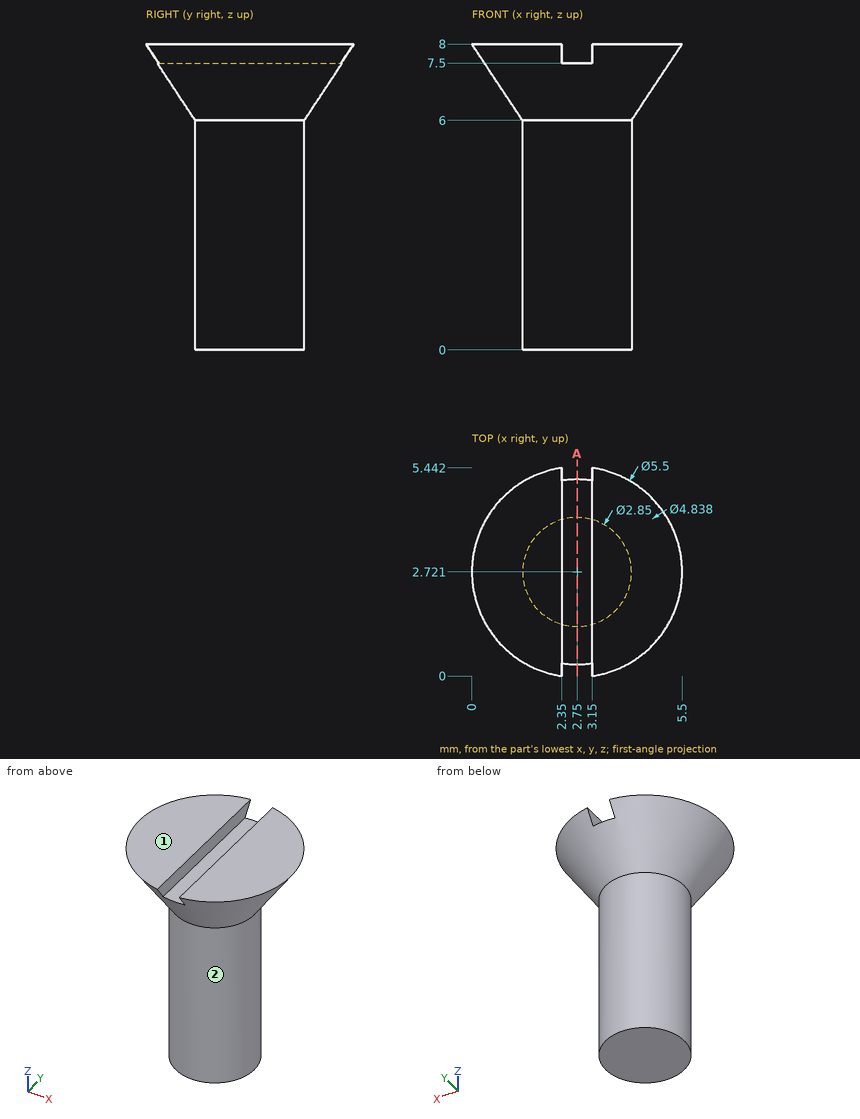
Geometry: see drawing. Coordinates: mm, zero at the bounding-box minimum. A direction names the side the tool comes from. Round coordinates to 2 decimals unless told otherwise and drop trailing zeros. Order: outer loops, then holes, each group sorted by start corner. A loop starts at its lowest first (then second) coordinate and runs counter-clockwise, first axis right, second up. Notation, with made-up numbers: (-34, 86) - (0, 86) arc R26 ccw to (0, 113) - close; hole circle Ø2 at (-32, -12). An arc over 180 degrees is marked (long way). One line per question, with ' | ' between items. Start each with the question number.
1) Contact query for a flat-ended pin moving along its axis: P1, Ø0.6, axis at y = 2.5, z = 7.5, coming from the +X side. Output: stop coordinate, or through.
2) Set-up query: the marked faces 1 and 2. Return all of +Z, -Z, +X, -X, +Y, -Y with unobstructed straight access to the full face (end or side cutting, diameter ignored); none if empty.
3) Cut plane A-A, the plane x = 2.75. Return the cut outline in (y, z) (1 decimal).
4) Ray query, probe 1 along X at (y, z) = (2.95, 7.25); probe 2 along Y at (x, z) = (2.2, 1) (1 decimal); probe 3 along X at (y, z) = (2.5, 6.5). Return the intervals inside material, ascending.
Worked out:
1) P1: stops at x = 5.36
2) face 1: +Z, +X, -X, +Y, -Y | face 2: -Z
3) outline: (0.3, 7.5) - (1.3, 6) - (1.3, 0) - (4.1, 0) - (4.1, 6) - (5.1, 7.5) - close
4) probe 1: x = 0.51 to 4.99 | probe 2: y = 1.4 to 4 | probe 3: x = 1.01 to 4.49
